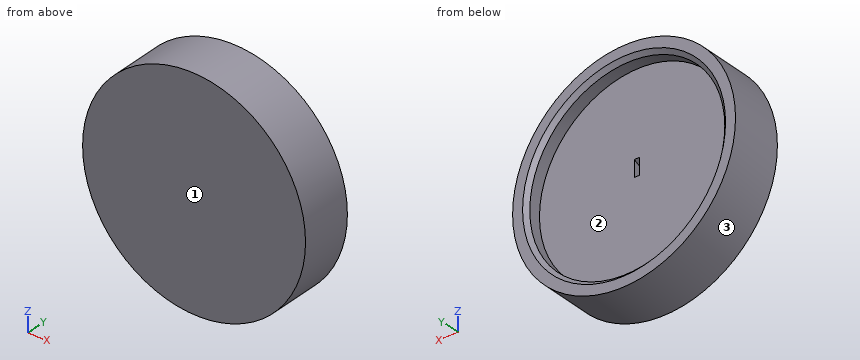
Autodesk Inventor part; units mm, degrees
ref_plane "YZ Plane" through (0, 0, 0) normal (1, 0, 0) x (0, 1, 0)
ref_plane "XZ Plane" through (0, 0, 0) normal (0, 1, 0) x (-1, 0, 0)
ref_plane "XY Plane" through (0, 0, 0) normal (0, 0, 1) x (1, 0, 0)
sketch "Sketch1" plane through (0, 0, 0) normal (0, 1, 0) x (-1, 0, 0)
  circle A0 centre (0, 0) radius 12.065 construction
  circle A1 centre (0, 0) radius 12.215
  dimension "d0" = 24.13
  dimension "d1" = 0.15
extrude "Extrusion1" add sketch "Sketch1" along normal mid plane 4.5
sketch "Sketch2" plane through (0, 0, 0) normal (1, 0, 0) x (0, 1, 0)
  line L0 (2.25, 1.7652) -> (-1.75, -0.1)
  line L1 (-1.75, -0.1) -> (2.25, -0.1)
  line L2 (2.25, -0.1) -> (2.25, 1.7652)
  line L3 (2.25, -12.215) -> (2.25, 12.215)
  line L4 (2.35, -0.2) -> (-2.2011, -0.2)
  line L5 (-2.2011, -0.2) -> (2.35, 1.9222)
  line L6 (2.35, 1.9222) -> (2.35, -0.2)
  point P0 (0, 0)
  dimension "d7" = 25
  dimension "d8" = 0.1
  dimension "d9" = 4
  dimension "d17" = 0.1
extrude "Extrusion2" cut sketch "Sketch2" against normal mid plane 0.65
sketch "Sketch3" plane through (0, 2.25, 0) normal (0, 1, 0) x (1, 0, 0)
  circle A0 centre (0, 0) radius 12.215
  circle A1 centre (0, 0) radius 13.965
  dimension "d12" = 1.75
extrude "Extrusion3" add sketch "Sketch3" along normal blind 2 and the other way blind 4.5
chamfer "Chamfer1" distance 0.5 angle 45 1 edges at (-12.215, 4.25, 0)
properties part number "Knife_Centering_Jig_LM6013" material "ABS Plastic"
Geometry: final body of the model. Coordinates: model frame, mm. Face numbers are marked on the shaded views. Give positions to 0.01 mm unless a question says otherwise; leave off trailing zeros. Write each loop counter-clockwise with the first axis right and the second up, starting at its lowest first coordinate (ties: lowest second). Pieces come first, ordered by that corner, then holes. Notation, with made-up numbers: (78, 24) -> (88, 24) arc R34 cw to (88, 56) -> close; hole circle Ø7 at (-3, -7). An arc over 180 degrees is marked (long way). Answer as a JSON object with one key per item and string values.
1. Ray query, probe 1 along X at (y, z) = (3.45, 0) (3 decimals); probe 2 along Y at (x, z) = (-10.5, -2.5). Return the intervals inside material, ascending. Write a range as from..to.
Ans:
{"probe 1": "x = -13.965..-12.215, 12.215..13.965", "probe 2": "y = -2.25..2.25"}
2. Cut plane B-B on y = -0.25. Output: boundary loops of the cut face in (x, z) (3 decimals), and give its area (3 significant figures).
Ans:
{"outline": "circle Ø27.93 at (0, 0); hole (-0.325, -0.2) -> (0.325, -0.2) -> (0.325, 0.71) -> (-0.325, 0.71) -> close", "area": "612 mm^2"}
3. Cut plane C-C on y = 3.25. Output: boundary loops of the cut face in (x, z) (3 decimals), and give its area (3 significant figures).
Ans:
{"outline": "circle Ø27.93 at (0, 0); hole circle Ø24.43 at (0, 0)", "area": "144 mm^2"}
4. Mould query, pull axis X, two halves, no side actions, for the marked faces 1, 2 and 3. Classes: pulls with the +X half, pulls with the -X half, needs draft (parallel to the pull), parting line crosses it, or undercut.
Ans:
{"face 1": "needs draft", "face 2": "undercut", "face 3": "parting line crosses it"}
5. Cut plane A-A on x = 0. Output: boundary loops of the cut face in (y, z) (3 decimals), and give its area (3 significant figures).
Ans:
{"outline": "(-2.25, -13.965) -> (4.25, -13.965) -> (4.25, -12.715) -> (3.75, -12.215) -> (2.25, -12.215) -> (2.25, -0.2) -> (-2.201, -0.2) -> (2.25, 1.876) -> (2.25, 12.215) -> (3.75, 12.215) -> (4.25, 12.715) -> (4.25, 13.965) -> (-2.25, 13.965) -> close", "area": "128 mm^2"}
6. Contact query for flat-ended pins moving along their axis: pin 1 (3 mm diameter, centred on y = -0.5, z = 4.5, fed in from +X); pin 2 (1 mm diameter, centred on y = 1, z = 1, fed in from -X); pin 3 (1.5 mm diameter, centred on y = 0, z = -5.5, fed in from +X). Output: stop coordinate, or through.
Ans:
{"pin 1": "stops at x = 13.64", "pin 2": "stops at x = -13.96", "pin 3": "stops at x = 13.13"}
